```python
from build123d import *

# Parameters (mm, degrees)
PAD_DEPTH = 2


with BuildPart() as part:
    # Sketch → Pad (new body)
    with BuildSketch(Plane.XY):
        with BuildLine():
            Line((0, 0), (15, 0))
            Line((15, 30), (15, 0))
            Line((14, 30), (15, 30))
            ThreePointArc((8, 36), (9.757359, 31.757359), (14, 30))
            Line((8, 200), (8, 36))
            Line((0, 200), (8, 200))
            Line((0, 200), (-8, 200))
            Line((-8, 200), (-8, 36))
            ThreePointArc((-14, 30), (-9.757359, 31.757359), (-8, 36))
            Line((-14, 30), (-15, 30))
            Line((-15, 30), (-15, 0))
            Line((0, 0), (-15, 0))
        make_face()
    pad = extrude(amount=PAD_DEPTH)

    # Mirrored: Pad across face of Pad
    add(pad.mirror(Plane(origin=(4, 200, 1), x_dir=(-1, 0, 0), z_dir=(0, 1, 0))))


solid = part.part
```
Model file for the job. Use its own axes, mm. Give positions to 0.01 mm unless a question says otherwise; leave off trailing zeros. Write each loop counter-clockwise with the first axis right and the second up, starting at its lowest first coordinate (ties: lowest second). Pieces come first, ordered by that corner, then holes. Notation, with made-up numbers: M 38,84 L 90,84 A15 cw 90,110 Z; hole C 81,18.25 d6. An arc over 180 degrees is marked long. Use a Markdown table: item, result.
1) Drill centre lines: line 1 (Y direction, x = 14, z = 0.7); line 2 (X direction, y = 336.5, z = 0.95); line 3 (Y direction, x = 9.25, z = 1.5). Where is each one in solid material? Low to high. Write a range as from..to.
Responses:
| item | result |
|---|---|
| line 1 | y = 0..30, 370..400 |
| line 2 | x = -8..8 |
| line 3 | y = 0..32.33, 367.67..400 |
2) Cut at B-B (y = 132.5). List the corners of the cut face in (x, z).
Responses:
| item | result |
|---|---|
| outline | M -8,0 L 8,0 L 8,2 L -8,2 Z |
3) Cut at A-A (z = 0.35). List the corners of the cut face in (x, y), and give its area (3 significant figures).
Responses:
| item | result |
|---|---|
| outline | M -15,0 L 15,0 L 15,30 L 14,30 A6 cw 8,36 L 8,364 A6 cw 14,370 L 15,370 L 15,400 L -15,400 L -15,370 L -14,370 A6 cw -8,364 L -8,36 A6 cw -14,30 L -15,30 Z |
| area | 7,270 mm2 |
